Could you check a few things on this model? Use its own coordinates, in mm. Face numbers are marked on the shaded views. A direction names the side the tool comes from. Give positions to 0.01 mm unless a question says otherwise; leave off trailing zeros. Loops run counter-clockwise (first coordinate to the right, second up) from the corner with the lowest first, then second, coordinate; pieces in that order, holes last. Notation, with made-up numbers: M 55,-4 L 101,-4 A13 cw 101,4 Z; hole C 19.25,30.5 d7. An arc over 180 degrees is marked long. Return JSON: item names as keys, results as strings. Group by question number.
1. For pin 1 (10 mm diameter, centred on x = 33, y = -36.5, fed in from -Z); pin 2 (10.5 mm diameter, centred on x = 48, y = 3, fed in from +Z); pin 3 (6 mm diameter, centred on x = -11, y = -18.5, fed in from +Z), each with a flat end and sliding along its axis, tell me the tip position at first contact or that it passes through.
2. For the marked faces 1, 2 and 3, which set-ups out of +Z, -Z, +X, -X, +Y, -Y let a thin tool reach every point of the face, with its end or its side?
3. If we section it at B-B (y = 2): Write out the boundary of the cut face in (x, z), plus the area to 3 significant figures.
4. If we section it at D-D (y = 48.5): Write out the boundary of the cut face in (x, z).
5. If we section it at C-C (x = 42): Write out the boundary of the cut face in (y, z), plus the area to 3 significant figures.
6. If we section it at A-A (z = 0): Write out the boundary of the cut face in (x, y).
7. Please list where these lines run through material, in increasing order: line 1 (X direction, y = 25.5, z = 0.5); line 2 (Y direction, x = 50.5, z = -3); line 3 (X direction, y = 13, z = 15).
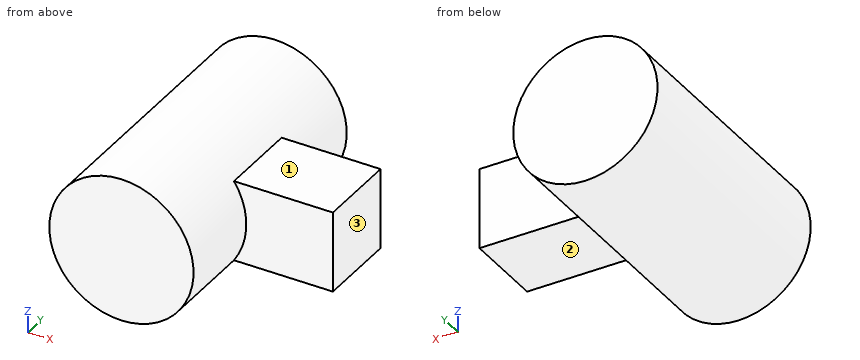
```python
from build123d import *

# Parameters (mm, degrees)
SKETCH1_R           = 31.75
BOSS_EXTRUDE1_DEPTH = 57.15
SKETCH2_W           = 35.56
SKETCH2_H           = 35.56
BOSS_EXTRUDE2_DEPTH = 69.85


with BuildPart() as part:
    # Sketch1 → Boss-Extrude1 (new, symmetric)
    with BuildSketch(Plane(origin=(0, 0, 0), x_dir=(1, 0, 0), z_dir=(0, 1, 0))):
        with Locations(Location((0, 0, 0), (0, 0, 270))):
            Circle(SKETCH1_R)
    extrude(amount=BOSS_EXTRUDE1_DEPTH, both=True)

    # Sketch2 → Boss-Extrude2 (add)
    with BuildSketch(Plane(origin=(0, 0, 0), x_dir=(0, 0, -1), z_dir=(1, 0, 0))):
        Rectangle(SKETCH2_W, SKETCH2_H)
    extrude(amount=BOSS_EXTRUDE2_DEPTH)


solid = part.part
```
Answer:
{
 "1": {"pin 1": "stops at z = -14.97", "pin 2": "stops at z = 17.78", "pin 3": "stops at z = 30.73"},
 "2": {"face 1": "+Z, +X, +Y, -Y", "face 2": "-Z, +X, +Y, -Y", "face 3": "+Z, -Z, +X, +Y, -Y"},
 "3": {"outline": "M 26.3,-17.78 L 69.85,-17.78 L 69.85,17.78 L 26.3,17.78 A31.75 ccw long Z", "area": "4,580 mm²"},
 "4": {"outline": "C 0,0 d63.5"},
 "5": {"outline": "M -17.78,-17.78 L 17.78,-17.78 L 17.78,17.78 L -17.78,17.78 Z", "area": "1,260 mm²"},
 "6": {"outline": "M -31.75,-57.15 L 31.75,-57.15 L 31.75,-17.78 L 69.85,-17.78 L 69.85,17.78 L 31.75,17.78 L 31.75,57.15 L -31.75,57.15 Z"},
 "7": {"line 1": "x = -31.75 to 31.75", "line 2": "y = -17.78 to 17.78", "line 3": "x = -27.98 to 69.85"}
}
